Geometry: see drawing. Coordinates: mm, zero at the bounding-box minimum. A direction names the side the tool comes from. Give positions to 0.01 mm unless a question says otherwise; leave off trailing zeros. Loops run counter-clockwise (first coordinate to the right, second up) from the corner with the lowest first, then second, coordinate; pieces in that order, holes last. Notation, with made-up numbers: M 78.5,22.5 L 112.5,22.5 A29 ccw 112.5,45.5 Z; hole C 26,-23 d4. An arc over 180 degrees is marked long. Return JSON: item names as keys, results as strings. Group by question number.
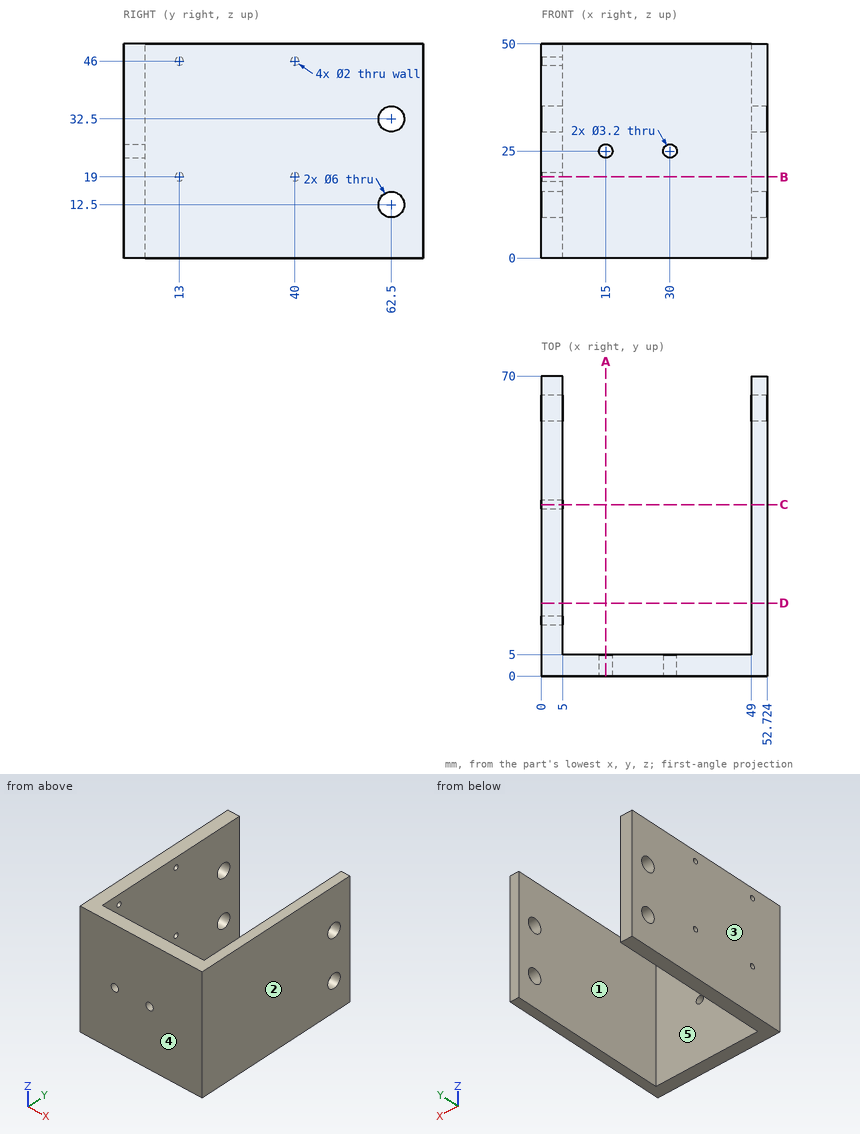
Item 1: First-contact query: pin 1 Ø4 at (x, z) = (10.5, 25) entering from -Y; pin 2 Ø1 at (x, z) = (14.5, 13) entering from +Y; pin 3 Ø1.6 at (y, z) = (40, 19) entering from -X. Flat tips, straight axial feed; report the tip coordinate or a pass-through.
Item 2: Material intervals for line 1 (Z direction, x = 2, y = 13); line 2 (Z direction, x = 50.3, y = 62.5); line 3 (X direction, y = 10, z = 30.5), sorted ascending. Write a range as from..to.
Item 3: Section D-D, the plane y = 17. Return loops of the section in (x, z), then the cut area to 3 significant figures.
Item 4: Section B-B, the plane z = 19. Return loops of the section in (x, y).
Item 5: Section C-C, the plane y = 40. Return loops of the section in (x, z).
Item 6: Pull-direction query (X, two-part tool) for the marked faces 3, 4 and 5; classes: pulls with the +X half, pulls with the -X half, needs draft (parallel to the pull), parting line crosses it, or undercut.
Item 7: Section A-A, the plane x = 15. Return loops of the section in (y, z).
Item 8: Reachability of the marked faces 1 and 2 from +Z, -Z, +X, -X, +Y, -Y: full face, straight path, thin tool, end or side. Return the list, or none.
Answer below:
{
 "1": {"pin 1": "y = 0", "pin 2": "y = 5", "pin 3": "x = 49"},
 "2": {"line 1": "0..18, 20..45, 47..50", "line 2": "0..9.5, 15.5..29.5, 35.5..50", "line 3": "0..5, 49..52.72"},
 "3": {"outline": "M 0,0 L 5,0 L 5,50 L 0,50 Z; M 49,0 L 52.72,0 L 52.72,50 L 49,50 Z", "area": "436 mm^2"},
 "4": {"outline": "M 0,0 L 52.72,0 L 52.72,70 L 49,70 L 49,5 L 5,5 L 5,12 L 0,12 Z; M 0,14 L 5,14 L 5,39 L 0,39 Z; M 0,41 L 5,41 L 5,70 L 0,70 Z"},
 "5": {"outline": "M 0,0 L 5,0 L 5,18 L 0,18 Z; M 0,20 L 5,20 L 5,45 L 0,45 Z; M 0,47 L 5,47 L 5,50 L 0,50 Z; M 49,0 L 52.72,0 L 52.72,50 L 49,50 Z"},
 "6": {"face 3": "pulls with the -X half", "face 4": "needs draft", "face 5": "undercut"},
 "7": {"outline": "M 0,0 L 5,0 L 5,23.4 L 0,23.4 Z; M 0,26.6 L 5,26.6 L 5,50 L 0,50 Z"},
 "8": {"face 1": "+Z, -Z, +Y", "face 2": "+Z, -Z, +X, +Y, -Y"}
}
